Design review of the part built by this model. Coordinates are the model's own, in mm. A direction names the side the tool comes from. Coordinates: 2 decimals unless noted, no trailing zeros. Order: outer loops, then holes, each group sorted by start corner. A loop starts at its lowest first (then second) coordinate and runs counter-clockwise, first axis right, second up. Notation, with made-up numbers: M 20,54.25 L 65,54.25 A13 ccw 65,75.25 Z; hole C -28,-23.75 d11. An arc over 180 degrees is marked long. Use CSV: the item, a comma, the result in double quotes.
```python
from build123d import *

# Parameters (mm, degrees)
SKETCH2_W           = 30
SKETCH2_H           = 8
CUT_EXTRUDE2_DEPTH  = 3
SKETCH3_W           = 42.75
SKETCH3_H           = 8
CUT_EXTRUDE3_DEPTH  = 3
CHAMFER1_SIZE       = 1
BOSS_EXTRUDE1_DEPTH = 6


with BuildPart() as part:
    # Sketch1 → Revolve1 (revolve)
    with BuildSketch(Plane(origin=(0, 0, 0), x_dir=(1, 0, 0), z_dir=(0, 1, 0))):
        Polygon((0, 0), (0, -10), (40, -10), (40, -12.5), (120, -12.5), (120, -17.5), (195, -17.5), (195, -15), (245, -15), (245, -12.5), (285, -12.5), (285, 0), align=None)
    revolve(axis=Axis((285, 0, 0), (-1, 0, 0)))

    # Sketch2 → Cut-Extrude2 (cut)
    with BuildSketch(Plane(origin=(0, 0, 15), x_dir=(-1, 0, 0), z_dir=(0, 0, -1))):
        with Locations((-220, 0)):
            Rectangle(SKETCH2_W, SKETCH2_H)
        with BuildLine():
            Line((-235, -4), (-235, 4))
            ThreePointArc((-235, 4), (-239, 0), (-235, -4))
        make_face()
        with BuildLine():
            Line((-205, -4), (-205, 4))
            ThreePointArc((-205, 4), (-201, 0), (-205, -4))
        make_face()
    extrude(amount=CUT_EXTRUDE2_DEPTH, mode=Mode.SUBTRACT)

    # Sketch3 → Cut-Extrude3 (cut)
    with BuildSketch(Plane.XY.offset(10)):
        with Locations((8.625, 0)):
            Rectangle(SKETCH3_W, SKETCH3_H)
        with BuildLine():
            Line((30, -4), (30, 4))
            ThreePointArc((30, 4), (34, 0), (30, -4))
        make_face()
    extrude(amount=-CUT_EXTRUDE3_DEPTH, mode=Mode.SUBTRACT)

    # Chamfer1
    chamfer1_edges = [part.edges().sort_by_distance(p)[0] for p in [
        (0, 0, -10),
        (285, 0, -12.5),
    ]]
    chamfer(chamfer1_edges, length=CHAMFER1_SIZE)

    # Sketch9 → Boss-Extrude1 (add)
    with BuildSketch(Plane.XY.offset(12)):
        with BuildLine():
            Line((235, 4), (205, 4))
            ThreePointArc((205, 4), (201, 0), (205, -4))
            Line((205, -4), (235, -4))
            ThreePointArc((235, -4), (239, 0), (235, 4))
        make_face()
    extrude(amount=BOSS_EXTRUDE1_DEPTH)


solid = part.part
```
(1) Clearance check with flat-ended pins moving along their axes: P1, Ø12, axis at x = 248.5, y = 9.5, coming from the +Z side; P2, Ø0.6, axis at x = 20, z = 8.5, coming from the -Y side; P3, Ø8, axis at x = 40, y = 6.5, coming from the -Z side. State where each tip first meets the part, or that it passes through.
The answers:
P1,"stops at z = 14.27"
P2,"stops at y = -5.72"
P3,"stops at z = -12.25"
(2) The part is to be moulded in two halves that separate along Y. For faces 4 (the face through (120, -8, -11)), 5 (the face through (17, 0, 7)), 6 (the face through (0.174, 0.351, -9.167)), say which applies: pulls with the +Y half, pulls with the -Y half, needs draft (parallel to the pull), parting line crosses it, or undercut.
The answers:
face 4,"needs draft"
face 5,"undercut"
face 6,"parting line crosses it"
(3) Add section C-C on x = 164. State the section outline as (y, z) points, and give its area (3 significant figures).
The answers:
outline,"C 0,0 d35"
area,"962 mm2"
(4) Wall thickness on probe 1 along X at (y, z) = (10.5, -1.5); probe 2 along X at (y, z) = (12.5, -8); probe 3 along Z at (x, y) = (110, 0.5): over which ranges is each line inside the solid? List them lowest first.
The answers:
probe 1,"x = 40 to 285"
probe 2,"x = 120 to 245"
probe 3,"z = -12.49 to 12.49"
(5) Add section A-A on z = 0. State the section outline as (x, y) points.
The answers:
outline,"M 0,-9 L 1,-10 L 40,-10 L 40,-12.5 L 120,-12.5 L 120,-17.5 L 195,-17.5 L 195,-15 L 245,-15 L 245,-12.5 L 284,-12.5 L 285,-11.5 L 285,11.5 L 284,12.5 L 245,12.5 L 245,15 L 195,15 L 195,17.5 L 120,17.5 L 120,12.5 L 40,12.5 L 40,10 L 1,10 L 0,9 Z"
(6) Add section D-D on x = 106.5. State the section outline as (y, z) points, and give its area (3 significant figures).
The answers:
outline,"C 0,0 d25"
area,"491 mm2"
(7) For faces 1 (the face through (264.773, 3.755, 11.923)), 2 (the face through (220, 0, 18)), 3 (the face through (40, 10.2, 0.1)), list the 3-axis set-ups (+Z, -Z, +X, -X, +Y, -Y) from which the entire face can be reached by the end or side of a thin tool; tool diameter is ignored.
The answers:
face 1,"+X"
face 2,"+Z, +X, -X, +Y, -Y"
face 3,"-X"
